from build123d import *

# Parameters (mm, degrees)
PAD002_DEPTH = 5.5
SKETCH005_R  = 4
PAD003_DEPTH = 26.1


with BuildPart() as part:
    # Sketch004 → Pad002 (new body)
    with BuildSketch(Plane.XY):
        Polygon((7.5055534995, 0), (3.7527767497, 6.5), (-3.7527767497, 6.5), (-7.5055534995, 0), (-3.7527767497, -6.5), (3.7527767497, -6.5), align=None)
    extrude(amount=PAD002_DEPTH)

    # Sketch005 (on Face8 of Pad002) → Pad003 (join)
    with BuildSketch(Plane.XY.offset(5.5)):
        Circle(SKETCH005_R)
    extrude(amount=PAD003_DEPTH)

    # Sketch006 → Groove (revolve, cut)
    with BuildSketch(Plane.XZ):
        Polygon((4, 31.6), (4.5, 31.6), (4, 31.1), align=None)
        Polygon((7.5055534995, 0), (6.3055534995, 0), (7.5055534995, -0.5), align=None)
        Polygon((7.5055534995, 5.5), (6.3055534995, 5.5), (7.5055534995, 6), align=None)
    revolve(axis=Axis((0, 0, 0), (0, 0, 1)), mode=Mode.SUBTRACT)


solid = part.part
Check sheet for the modelled part. Datum: model origin and axes. Units: mm. A direction names the side the tool comes from. Give positions to 0.01 mm unless a question says otherwise; leave off trailing zeros. Loops run counter-clockwise (first coordinate to the right, second up) from the corner with the lowest first, then second, coordinate; pieces in that order, holes last. Notation, with made-up numbers: M 88.5,-27 L 111.5,-27 A9 ccw 111.5,-21 Z; hole C 57.25,49.5 d11. An arc over 180 degrees is marked long. Return JSON: item names as keys, results as strings. Group by question number.
1. Cross-section at B-B on y = -3.5. Record the boundary of the cut face in (x, z).
2. Cross-section at C-C on z = 8. Record the boundary of the cut face in (x, y), plus the area to 3 significant figures.
3. Go/stop test with flat-tipped pins: pin 1 (3 mm diameter, centred on x = 2.5, z = 25.5, fed in from +Y); pin 2 (8 mm diameter, centred on x = -1.5, z = 20, fed in from -Y); pin 3 (6 mm diameter, centred on x = -5, z = 10.5, fed in from +Y). Record where each tip stops, or that it passes through.
4. Thickness scan on L1, parallel to Z at x = 4.75, y = -3.25; L2, parallel to X at y = 0.25, z = 12; L3, parallel to X at y = -1.75, z = 2.5. Record the ranges inside material, lowest first.
5. Cross-section at A-A on x = 0. Record the boundary of the cut face in (y, z).
6. Cross-section at D-D on x = -6.25. Record the boundary of the cut face in (y, z).
7. Tool access check on faces 1 (the flat face through (0, 0, 0)), 2 (the cylindrical face through (-0.867, -3.905, 18.367)). Record the directions out of +Z, -Z, +X, -X, +Y, -Y that give a thin tool (end or side, any length) a straight path to the whole face; none if there is none.
Return value:
{
 "1": {"outline": "M -5.48,0 L 5.48,0 L 5.48,5.5 L 1.94,5.5 L 1.94,31.6 L -1.94,31.6 L -1.94,5.5 L -5.48,5.5 Z"},
 "2": {"outline": "C 0,0 d8", "area": "50.3 mm^2"},
 "3": {"pin 1": "y = 3.87", "pin 2": "y = -4", "pin 3": "y = 3.46"},
 "4": {"L1": "0 to 5.5", "L2": "-3.99 to 3.99", "L3": "-6.5 to 6.5"},
 "5": {"outline": "M -6.5,0 L 6.5,0 L 6.5,5.5 L 4,5.5 L 4,31.6 L -4,31.6 L -4,5.5 L -6.5,5.5 Z"},
 "6": {"outline": "M -2.17,0 L 2.17,0 L 2.17,5.5 L -2.17,5.5 Z"},
 "7": {"face 1": "-Z, +X, -X, +Y, -Y", "face 2": "+Z"}
}
